Check sheet for the modelled part. Datum: model origin and axes. Units: mm. Face numbers are marked on the shaded views. A direction names the side the tool comes from. Give positions to 0.01 mm unless a question says otherwise; leave off trailing zeros. Order: outer loops, then holes, each group sorted by start corner. A loop starts at its lowest first (then second) coordinate and runs counter-clockwise, first axis right, second up. Notation, with made-up numbers: (-1.75, -19.5) -> (36.25, -19.5) arc R8 ccw to (36.25, -14.5) -> close; hole circle Ø3 at (30.5, 62.5). An arc over 180 degrees is marked (long way). Answer in a Markdown table with one row per item. Add a question column.
(1) Release check for a two-part mould opening along X. For the marked faces 3, 4 and 5 record: released by +X, released by -X, zero draft, split by the parting line, or undercut.
(2) Cross-section at C-C (x = 40). Record the cut outline in (y, z).
(3) Set-up check for the marked faces 1 and 2: record each of +Z, -Z, +X, -X, +Y, -Y from which the full face is reachable in a straight line by a thin tool's end or side.
(4) Go/stop test with a flat-tipped pin: pin 1 (1.5 mm diameter, centred on x = -3, y = -11, fed in from +Z). Record where the tip stops, or that it passes through.
(5) Cross-section at B-B (z = 53). Record the cut outline in (x, y), then the cut area to 3 significant figures.
(6) Thickness scan on L1, parallel to X at y = 13.5, z = 0.95; L2, parallel to Y at x = -28, z = 2.2; L3, parallel to Y at x = -29, z = 9.5. Record the ranges inside material, lowest first. Write a range as [from, to].
(7) Cross-section at A-A (z = 72). Record the cut outline in (x, y).
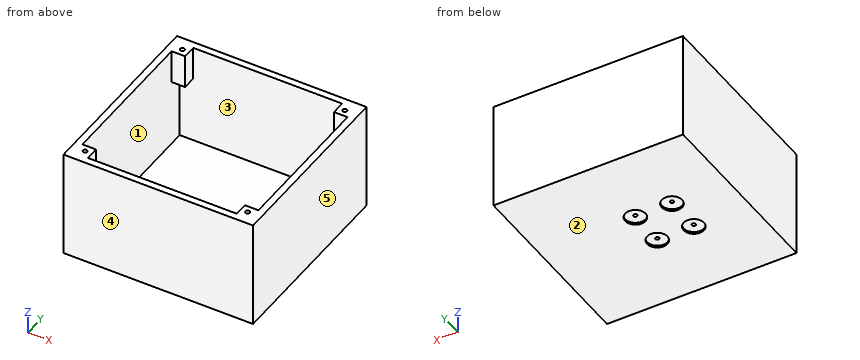
```python
from build123d import *

# Parameters (mm, degrees)
F0_W     = 140
F0_H     = 140
F0_W_2   = 130
F0_H_2   = 130
F1_DEPTH = 80
F2_W     = 140
F2_H     = 140
F3_DEPTH = 5
F4_R     = 1.4
F5_DEPTH = 5
F6_R     = 7.5
F7_DEPTH = 1.5
F8_W     = 10
F8_H     = 10
F8_R     = 1.6
F9_DEPTH = 25


with BuildPart() as f1:
    # F0 (on Top) → F1 (new body)
    with BuildSketch(Plane.XY):
        Rectangle(F0_W, F0_H)
        Rectangle(F0_W_2, F0_H_2, mode=Mode.SUBTRACT)
    extrude(amount=F1_DEPTH)

    # F2 (on face) → F3 (join)
    with BuildSketch(Plane(origin=(0, 0, 0), x_dir=(1, 0, 0), z_dir=(0, 0, -1))):
        Rectangle(F2_W, F2_H)
    extrude(amount=-F3_DEPTH)

    # F4 (on face) → F5 (cut, through all)
    with BuildSketch(Plane.XY.offset(5)):
        with Locations((-1, 13.5)):
            Circle(F4_R)
        with Locations((-28, 13.5)):
            Circle(F4_R)
        with Locations((-1, -13.5)):
            Circle(F4_R)
        with Locations((-28, -13.5)):
            Circle(F4_R)
    extrude(amount=-F5_DEPTH, mode=Mode.SUBTRACT)

    # F6 (on face) → F7 (cut)
    with BuildSketch(Plane(origin=(0, 0, 0), x_dir=(1, 0, 0), z_dir=(0, 0, -1))):
        with Locations((-28, 13.5)):
            Circle(F6_R)
        with Locations((-1, 13.5)):
            Circle(F6_R)
        with Locations((-28, -13.5)):
            Circle(F6_R)
        with Locations((-1, -13.5)):
            Circle(F6_R)
    extrude(amount=-F7_DEPTH, mode=Mode.SUBTRACT)

    # F8 (on face) → F9 (join)
    with BuildSketch(Plane.XY.offset(80)):
        with Locations((-60, 60)):
            Rectangle(F8_W, F8_H)
        with Locations((-60, 60)):
            Circle(F8_R, mode=Mode.SUBTRACT)
        with Locations((60, 60)):
            Rectangle(F8_W, F8_H)
        with Locations((60, 60)):
            Circle(F8_R, mode=Mode.SUBTRACT)
        with Locations((-60, -60)):
            Rectangle(F8_W, F8_H)
        with Locations((-60, -60)):
            Circle(F8_R, mode=Mode.SUBTRACT)
        with Locations((60, -60)):
            Rectangle(F8_W, F8_H)
        with Locations((60, -60)):
            Circle(F8_R, mode=Mode.SUBTRACT)
    extrude(amount=-F9_DEPTH)


solid = f1.part
```
Answer below:
| question | item | result |
|---|---|---|
| 1 | face 3 | undercut |
| 1 | face 4 | zero draft |
| 1 | face 5 | released by +X |
| 2 | outline | (-70, 0) -> (70, 0) -> (70, 80) -> (65, 80) -> (65, 5) -> (-65, 5) -> (-65, 80) -> (-70, 80) -> close |
| 3 | face 1 | none |
| 3 | face 2 | -Z, +X, -X, +Y, -Y |
| 4 | pin 1 | stops at z = 5 |
| 5 | outline | (-70, -70) -> (70, -70) -> (70, 70) -> (-70, 70) -> close; hole (-65, -65) -> (65, -65) -> (65, 65) -> (-65, 65) -> close |
| 5 | area | 2,700 mm² |
| 6 | L1 | x = [-70, -35.5], [-20.5, -8.5], [6.5, 70] |
| 6 | L2 | y = [-70, -14.9], [-12.1, 12.1], [14.9, 70] |
| 6 | L3 | y = [-70, -65], [65, 70] |
| 7 | outline | (-70, -70) -> (70, -70) -> (70, 70) -> (-70, 70) -> close; hole (-65, -55) -> (-55, -55) -> (-55, -65) -> (55, -65) -> (55, -55) -> (65, -55) -> (65, 55) -> (55, 55) -> (55, 65) -> (-55, 65) -> (-55, 55) -> (-65, 55) -> close; hole circle Ø3.2 at (-60, -60); hole circle Ø3.2 at (-60, 60); hole circle Ø3.2 at (60, -60); hole circle Ø3.2 at (60, 60) |
